Geometry: see drawing. Coordinates: mm, zero at the bounding-box minimum. Coordinates: 2 decimals unless noted, no trailing zeros. Loops run counter-clockwise (first coordinate to the right, second up) from the corner with the lowest first, then second, coordinate; pieces in that order, holes last. Notation, with made-up numbers: (-37, 81.5) - (-22, 81.5) arc R14 ccw to (-22, 91.5) - close; hole circle Ø6 at (30, 70.5). An arc over 180 degrees is marked (long way). Write item = value, one per line. Start each with the question number.
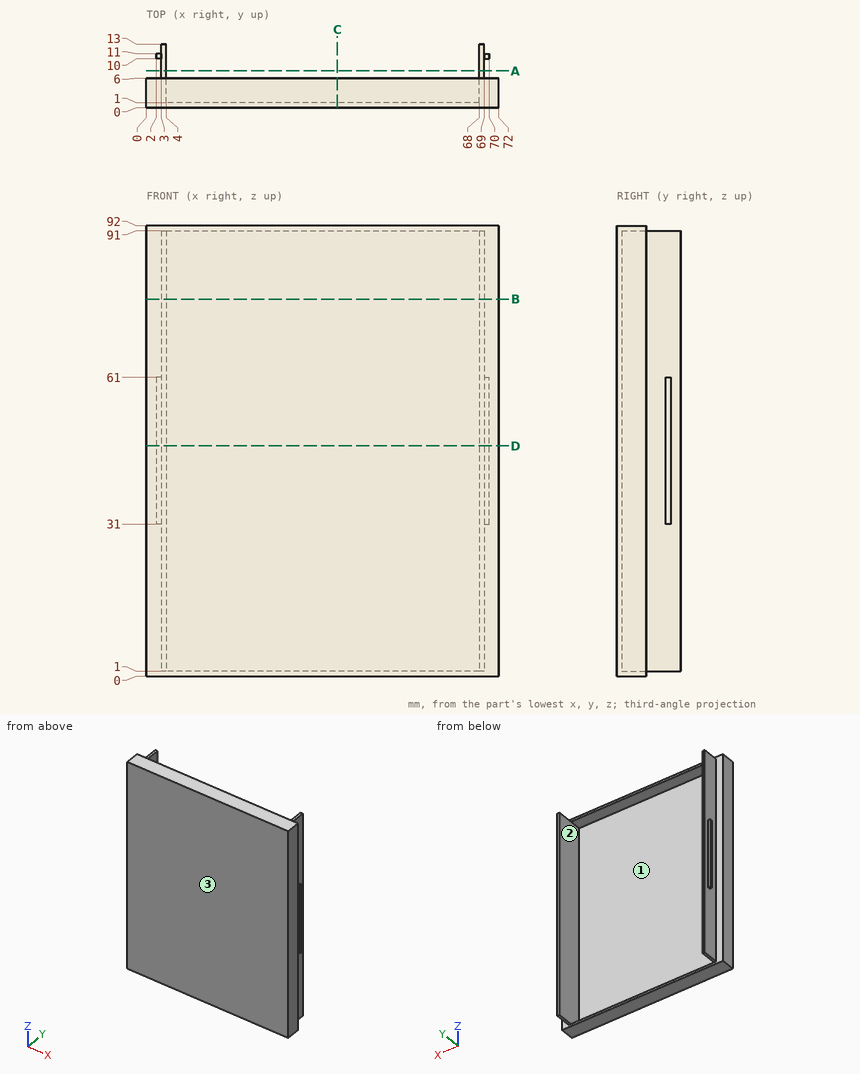
Item 1: Cut plane A-A (y = 7.5). Return the cut outline in (x, z), then the cut area to 3 significant figures.
Item 2: First-contact query: pin 1 (0.8 mm diameter, centred on x = 2.5, y = 10.5, fed in from -Z); pin 2 (1.1 mm diameter, centred on x = 68.5, y = 10.5, fed in from +Z); pin 3 (8 mm diameter, centred on x = 21, z = 57, fed in from +Y). Flat tips, straight axial feed; report the tip coordinate or a pass-through.
Item 3: Cut plane C-C (x = 39). Return the cut outline in (y, z).
Item 4: Cut plane B-B (z = 77). Return the cut outline in (x, y).
Item 5: Draft query along Z for the marked faces 1, 2 and 3. Return one class per face: released by +Z, released by -Z, zero draft, split by the parting line, or undercut.
Item 6: Material intervals for L1, parallel to X at y = 9.75, z = 8; L2, parallel to Z at x = 55.5, y = 2.75; L3, parallel to X at y = 10.75, z = 59, sorted ascending. Write a range as [from, to].
Item 7: Cut plane D-D (z = 47). Return the cut outline in (x, y).
Responses:
q1.outline = (3, 1) - (4, 1) - (4, 91) - (3, 91) - close; (68, 1) - (69, 1) - (69, 91) - (68, 91) - close
q1.area = 180 mm2
q2.pin_1 = 31
q2.pin_2 = 91
q2.pin_3 = 1
q3.outline = (0, 0) - (6, 0) - (6, 1) - (1, 1) - (1, 91) - (6, 91) - (6, 92) - (0, 92) - close
q4.outline = (0, 0) - (72, 0) - (72, 6) - (69, 6) - (69, 13) - (68, 13) - (68, 1) - (4, 1) - (4, 13) - (3, 13) - (3, 6) - (0, 6) - close
q5.face_1 = undercut
q5.face_2 = undercut
q5.face_3 = zero draft
q6.L1 = [3, 4], [68, 69]
q6.L2 = [0, 1], [91, 92]
q6.L3 = [2, 4], [68, 70]
q7.outline = (0, 0) - (72, 0) - (72, 6) - (69, 6) - (69, 10) - (70, 10) - (70, 11) - (69, 11) - (69, 13) - (68, 13) - (68, 1) - (4, 1) - (4, 13) - (3, 13) - (3, 11) - (2, 11) - (2, 10) - (3, 10) - (3, 6) - (0, 6) - close
